Autodesk Inventor part; units mm, degrees
ref_plane "YZ Plane" through (0, 0, 0) normal (1, 0, 0) x (0, 1, 0)
ref_plane "XZ Plane" through (0, 0, 0) normal (0, 1, 0) x (-1, 0, 0)
ref_plane "XY Plane" through (0, 0, 0) normal (0, 0, 1) x (1, 0, 0)
sketch "스케치1" plane through (0, 0, 0) normal (0, 0, 1) x (1, 0, 0)
  circle A0 centre (11, 3) radius 1.35
  circle A1 centre (-5, 3) radius 1.35
  line L0 (0, 0) -> (6, 0)
  line L1 (6, 0) -> (6, 6)
  line L2 (0, 6) -> (6, 6)
  line L3 (0, 0) -> (0, 6)
  circle A2 centre (11, -53.9) radius 1.35
  circle A3 centre (-5, -53.9) radius 1.35
  line L4 (0, -56.9) -> (6, -56.9)
  line L5 (6, -56.9) -> (6, -50.9)
  line L6 (0, -50.9) -> (6, -50.9)
  line L7 (0, -56.9) -> (0, -50.9)
  line L8 (21, 16) -> (-35, 16)
  line L9 (-35, 16) -> (-35, -78)
  line L10 (-35, -78) -> (21, -78)
  line L11 (21, -78) -> (21, 16)
  circle A4 centre (11, 3) radius 1.35
  circle A5 centre (-5, 3) radius 1.35
  circle A6 centre (11, -53.9) radius 1.35
  circle A7 centre (-5, -53.9) radius 1.35
  line L12 (-0.05, 6.05) -> (6.05, 6.05)
  line L13 (6.05, 6.05) -> (6.05, -0.05)
  line L14 (6.05, -0.05) -> (-0.05, -0.05)
  line L15 (-0.05, -0.05) -> (-0.05, 6.05)
  line L16 (-0.05, 6.05) -> (6.05, -0.05) construction
  line L17 (6.05, 6.05) -> (-0.05, -0.05) construction
  line L18 (-0.05, -50.85) -> (6.05, -50.85)
  line L19 (6.05, -50.85) -> (6.05, -56.95)
  line L20 (6.05, -56.95) -> (-0.05, -56.95)
  line L21 (-0.05, -56.95) -> (-0.05, -50.85)
  line L22 (-0.05, -50.85) -> (6.05, -56.95) construction
  line L23 (6.05, -50.85) -> (-0.05, -56.95) construction
  point P0 (3, 3)
  point P1 (3, -53.9)
  dimension "d0" = 56
  dimension "d1" = 94
  dimension "d2" = 2.7
  dimension "d3" = 2.7
  dimension "d4" = 2.7
  dimension "d5" = 2.7
  dimension "d6" = 6.1
  dimension "d7" = 6.1
  dimension "d8" = 6.1
  dimension "d9" = 6.1
extrude "돌출1" add sketch "스케치1" along normal blind 6 contours L11 L10 L9 L8
fillet "모깎기1" radius 2 4 edges at (-35, 16, 3) (21, 16, 3) (-35, -78, 3) (21, -78, 3)
sketch "스케치3" plane through (0, 0, 6) normal (0, 0, 1) x (1, 0, 0)
  line L0 (-0.05, 6.05) -> (6.05, 6.05)
  line L1 (6.05, 6.05) -> (6.05, -0.05)
  line L2 (-0.05, -0.05) -> (-0.05, 6.05)
  line L3 (6.05, -0.05) -> (-0.05, -0.05)
  line L4 (-2.05, -0.05) -> (8.05, -0.05)
  line L5 (8.05, -0.05) -> (8.05, 6.05)
  line L6 (8.05, 6.05) -> (-2.05, 6.05)
  line L7 (-2.05, 6.05) -> (-2.05, -0.05)
  line L8 (-2.05, -0.05) -> (8.05, 6.05) construction
  line L9 (8.05, -0.05) -> (-2.05, 6.05) construction
  line L10 (-0.05, -50.85) -> (6.05, -50.85)
  line L11 (6.05, -50.85) -> (6.05, -56.95)
  line L12 (-0.05, -56.95) -> (-0.05, -50.85)
  line L13 (6.05, -56.95) -> (-0.05, -56.95)
  line L14 (-2.05, -56.95) -> (8.05, -56.95)
  line L15 (8.05, -56.95) -> (8.05, -50.85)
  line L16 (8.05, -50.85) -> (-2.05, -50.85)
  line L17 (-2.05, -50.85) -> (-2.05, -56.95)
  line L18 (-2.05, -56.95) -> (8.05, -50.85) construction
  line L19 (8.05, -56.95) -> (-2.05, -50.85) construction
  point P0 (0, 0)
  point P1 (3, 3)
  point P2 (3, -53.9)
  dimension "d13" = 10.1
  dimension "d14" = 10.1
  dimension "d15" = 6.1
extrude "돌출2" cut sketch "스케치3" against normal blind 10
sketch "스케치4" plane through (0, 0, 6) normal (0, 0, 1) x (1, 0, 0)
  line L0 (-2.05, 6.05) -> (8.05, 6.05)
  line L1 (8.05, 6.05) -> (8.05, -0.05)
  line L2 (-2.05, -0.05) -> (-2.05, 6.05)
  line L3 (8.05, -0.05) -> (-2.05, -0.05)
  line L4 (-2.05, -50.85) -> (8.05, -50.85)
  line L5 (8.05, -50.85) -> (8.05, -56.95)
  line L6 (8.05, -56.95) -> (-2.05, -56.95)
  line L7 (-2.05, -56.95) -> (-2.05, -50.85)
  circle A0 centre (-2.05, 6.05) radius 1
  circle A1 centre (8.05, 6.05) radius 1
  circle A2 centre (8.05, -0.05) radius 1
  circle A3 centre (-2.05, -0.05) radius 1
  circle A4 centre (-2.05, -50.85) radius 1
  circle A5 centre (8.05, -50.85) radius 1
  circle A6 centre (8.05, -56.95) radius 1
  circle A7 centre (-2.05, -56.95) radius 1
  point P0 (0, 0)
  dimension "d18" = 2
  dimension "d19" = 2
  dimension "d20" = 2
  dimension "d21" = 2
  dimension "d22" = 2
  dimension "d23" = 2
  dimension "d24" = 2
  dimension "d25" = 2
extrude "돌출3" cut sketch "스케치4" against normal blind 10 contours L2 A0 L0 | L0 A0 L2 | A1 L1 L0 | L0 L1 A1 | A3 L3 L2 | L2 L3 A3 | A2 L3 L1 | L1 L3 A2 | L7 A4 L4 | L4 A4 L7 | A5 L5 L4 | L4 L5 A5 | A7 L6 L7 | L7 L6 A7 | A6 L6 L5 | L5 L6 A6
sketch "스케치5" plane through (0, 0, 6) normal (0, 0, 1) x (1, 0, 0)
  line L0 (-1.05, 6.05) -> (7.05, 6.05)
  line L1 (8.05, 5.05) -> (8.05, 0.95)
  circle A0 centre (-2.8, -9.5) radius 1.35
  circle A1 centre (8.8, -9.5) radius 1.35
  circle A2 centre (-2.8, -39.5) radius 1.35
  circle A3 centre (8.8, -39.5) radius 1.35
  point P0 (0, 0)
  dimension "d32" = 2.7
  dimension "d33" = 2.7
  dimension "d34" = 2.7
  dimension "d35" = 2.7
extrude "돌출4" cut sketch "스케치5" against normal blind 10
sketch "스케치6" plane through (0, 0, 6) normal (0, 0, 1) x (1, 0, 0)
  line L0 (-11.1766, 9.439) -> (14.0881, 9.439)
  line L1 (14.0881, 9.439) -> (14.0881, -4.9308)
  line L2 (14.0881, -4.9308) -> (-11.1766, -4.9308)
  line L3 (-11.1766, -4.9308) -> (-11.1766, 9.439)
  line L4 (-9.3673, -48.6772) -> (15.6068, -48.6772)
  line L5 (15.6068, -48.6772) -> (15.6068, -64.9024)
  line L6 (15.6068, -64.9024) -> (-9.3673, -64.9024)
  line L7 (-9.3673, -64.9024) -> (-9.3673, -48.6772)
  point P0 (0, 0)
extrude "돌출5" add sketch "스케치6" against normal blind 6
properties part number "foot_ver2" material "PMMA 플라스틱"
Input: part model. Units: mm. Frame: model coordinates. Coordinates: 2 decimals unless noted, no trailing zeros. Write each loop counter-clockwise with the first axis right and the second up, starting at its lowest first coordinate (ties: lowest second). Pieces come first, ordered by that corner, then holes.
1) Material intervals for line 1 along Y through (x, z) = (-2.8, 4.2), sorted ascending.
2) Section B-B on x = -2.8. Output: boundary loops of the cut face in (y, z).
3) Mould query, pull axis X, two halves, no side actions, for faces 1 (the cylindrical face through (20.4, -77.43, 3.04)), 2 (the flat face through (-7, 16, 3)), 3 (the cylindrical face through (-2.976, -8.161, 3.042)). Classes: pulls with the +X half, pulls with the -X half, needs draft (parallel to the pull), parting line crosses it, or undercut.
4) Section A-A on y = -9.5. Output: boundary loops of the cut face in (x, z), and give its area (3 significant figures).
5) Pin query (flat end, axial travel): pin 1 Ø1.6 at (x, y) = (8.8, -9.5) entering from -Z. Return the tip coordinate at first contact, or that it passes through.
Check result:
1. line 1: y = -78 to -40.85, -38.15 to -10.85, -8.15 to 16
2. outline: (-78, 0) - (-40.85, 0) - (-40.85, 6) - (-78, 6) - close; (-38.15, 0) - (-10.85, 0) - (-10.85, 6) - (-38.15, 6) - close; (-8.15, 0) - (16, 0) - (16, 6) - (-8.15, 6) - close
3. face 1: pulls with the +X half
3. face 2: needs draft
3. face 3: undercut
4. outline: (-35, 0) - (-4.15, 0) - (-4.15, 6) - (-35, 6) - close; (-1.45, 0) - (7.45, 0) - (7.45, 6) - (-1.45, 6) - close; (10.15, 0) - (21, 0) - (21, 6) - (10.15, 6) - close
4. area: 304 mm2
5. pin 1: passes through
